```python
from build123d import *

# Parameters (mm, degrees)
SKETCH1_R               = 49.53
EXTRUDE1_DEPTH          = 1.5875
SKETCH2_R               = 2.06375
EXTRUDE2_DEPTH          = 10
MIRROR3_COPY_1_SKETCH_R = 2.06375
MIRROR3_COPY_1_DEPTH    = 10


with BuildPart() as part:
    # Sketch1 → Extrude1 (new body)
    with BuildSketch(Plane(origin=(0, 0, 0), x_dir=(1, 0, 0), z_dir=(0, 1, 0))):
        with Locations(Location((0, 0, 0), (0, 0, 270))):
            Circle(SKETCH1_R)
    extrude(amount=EXTRUDE1_DEPTH)

    # Sketch2 → Extrude2 (cut)
    with BuildSketch(Plane(origin=(0, 1.5875, 0), x_dir=(-1, 0, 0), z_dir=(0, 1, 0))):
        with Locations(Location((-26, -30, 0), (0, 0, 90))):
            Circle(SKETCH2_R)
    extrude2 = extrude(amount=-EXTRUDE2_DEPTH, mode=Mode.SUBTRACT)

    # Mirror1: Extrude2 across plane
    add(extrude2.mirror(Plane(origin=(0, 0, 0), x_dir=(0, 0, 1), z_dir=(1, 0, 0))), mode=Mode.SUBTRACT)

    # Mirror3: Extrude2 across plane
    add(extrude2.mirror(Plane.XY), mode=Mode.SUBTRACT)

    # Mirror3 copy 1 sketch → Mirror3 copy 1 (cut)
    with BuildSketch(Plane(origin=(0, 1.5875, 0), x_dir=(1, 0, 0), z_dir=(0, 1, 0))):
        with Locations(Location((-26, -30, 0), (0, 0, 90))):
            Circle(MIRROR3_COPY_1_SKETCH_R)
    extrude(amount=-MIRROR3_COPY_1_DEPTH, mode=Mode.SUBTRACT)


solid = part.part
```
Here's how the part is built. I have some questions about the finished solid (model axes, mm). Coordinates: 2 decimals unless noted, no trailing zeros. Order: outer loops, then holes, each group sorted by start corner. A loop starts at its lowest first (then second) coordinate and runs counter-clockwise, first axis right, second up. Notation, with made-up numbers: (39, 86.5) - (90, 86.5) arc R19 ccw to (90, 113.5) - close; hole circle Ø9 at (47.5, 71.5). An arc over 180 degrees is marked (long way). One line per question, with ' | ' between items. Start each with the question number.
1. I'm going to push a flat-ended pin straight in: pin 1 Ø4.5 at (x, z) = (-26, 30) entering from -Y. Where does the tip first touch, or does it pass through?
2. If we section it at B-B (y = 1.3): Write out the boundary of the cut face in (x, z), and give its area (3 significant figures).
3. If we section it at A-A (x = -26): Write out the boundary of the cut face in (y, z), and give its area (3 significant figures).
4. If we mould it in two halves opening along X, with no side actions, what happens to faces 1 (the cylindrical face through (-26.09, 0.8, 32.06)), 2 (the cylindrical face through (14.88, 0.78, 47.24)), 3 (the flat face through (1, 1.588, -1))? For each: released by +X, released by -X, zero draft, split by the parting line, or undercut.
5. Please list where these lines run through material, in increasing order: line 1 along Z through (x, y) = (-26, 1.1); line 2 along Z through (x, y) = (26.5, 1.45); line 3 along X through (y, z) = (1.3, -30). Write a range as [from, to].
6. If we section it at C-C (z = -30): Write out the boundary of the cut face in (x, y), and give its area (3 significant figures).
7. If we section it at D-D (z = 19): Write out the boundary of the cut face in (x, y), and give its area (3 significant figures).
Model answer:
1) pin 1: stops at y = 0
2) outline: circle Ø99.06 at (0, 0); hole circle Ø4.13 at (-26, -30); hole circle Ø4.13 at (-26, 30); hole circle Ø4.13 at (26, -30); hole circle Ø4.13 at (26, 30) | area: 7,650 mm²
3) outline: (0, -42.16) - (1.59, -42.16) - (1.59, -32.06) - (0, -32.06) - close; (0, -27.94) - (1.59, -27.94) - (1.59, 27.94) - (0, 27.94) - close; (0, 32.06) - (1.59, 32.06) - (1.59, 42.16) - (0, 42.16) - close | area: 121 mm²
4) face 1: undercut | face 2: split by the parting line | face 3: zero draft
5) line 1: z = [-42.16, -32.06], [-27.94, 27.94], [32.06, 42.16] | line 2: z = [-41.84, -32], [-28, 28], [32, 41.84] | line 3: x = [-39.41, -28.06], [-23.94, 23.94], [28.06, 39.41]
6) outline: (-39.41, 0) - (-28.06, 0) - (-28.06, 1.59) - (-39.41, 1.59) - close; (-23.94, 0) - (23.94, 0) - (23.94, 1.59) - (-23.94, 1.59) - close; (28.06, 0) - (39.41, 0) - (39.41, 1.59) - (28.06, 1.59) - close | area: 112 mm²
7) outline: (-45.74, 0) - (45.74, 0) - (45.74, 1.59) - (-45.74, 1.59) - close | area: 145 mm²
